from build123d import *

# Parameters (mm, degrees)
AUFSATZ_LINEAR_AUSTRAGEN1_DEPTH = 20
AUFSATZ_LINEAR_AUSTRAGEN2_DEPTH = 10
SKIZZE3_R                       = 25
SCHNITT_LINEAR_AUSTRAGEN1_DEPTH = 15


with BuildPart() as part:
    # Skizze1 → Aufsatz-Linear austragen1 (new body)
    with BuildSketch(Plane.XY):
        with BuildLine():
            Line((-0.330334949, 95.09360025), (369.669665051, 95.09360025))
            ThreePointArc((369.669665051, 95.09360025), (405.02500411, 80.448939309), (419.669665051, 45.09360025))
            Line((419.669665051, 45.09360025), (419.669665051, -224.90639975))
            ThreePointArc((419.669665051, -224.90639975), (405.02500411, -260.26173881), (369.669665051, -274.90639975))
            Line((369.669665051, -274.90639975), (-0.330334949, -274.90639975))
            ThreePointArc((-0.330334949, -274.90639975), (-35.685674008, -260.26173881), (-50.330334949, -224.90639975))
            Line((-50.330334949, -224.90639975), (-50.330334949, 45.09360025))
            ThreePointArc((-50.330334949, 45.09360025), (-35.685674008, 80.448939309), (-0.330334949, 95.09360025))
        make_face()
        with BuildLine():
            Line((-0.330334949, 85.09360025), (369.669665051, 85.09360025))
            ThreePointArc((369.669665051, 85.09360025), (397.953936298, 73.377871497), (409.669665051, 45.09360025))
            Line((409.669665051, 45.09360025), (409.669665051, -224.90639975))
            ThreePointArc((409.669665051, -224.90639975), (397.953936298, -253.190670998), (369.669665051, -264.90639975))
            Line((369.669665051, -264.90639975), (-0.330334949, -264.90639975))
            ThreePointArc((-0.330334949, -264.90639975), (-28.614606196, -253.190670998), (-40.330334949, -224.90639975))
            Line((-40.330334949, -224.90639975), (-40.330334949, 45.09360025))
            ThreePointArc((-40.330334949, 45.09360025), (-28.614606196, 73.377871497), (-0.330334949, 85.09360025))
        make_face(mode=Mode.SUBTRACT)
    extrude(amount=AUFSATZ_LINEAR_AUSTRAGEN1_DEPTH)

    # Skizze2 → Aufsatz-Linear austragen2 (add)
    with BuildSketch(Plane.XY):
        with BuildLine():
            Line((-0.330334949, -264.90639975), (369.669665051, -264.90639975))
            ThreePointArc((369.669665051, -264.90639975), (397.953936298, -253.190670998), (409.669665051, -224.90639975))
            Line((409.669665051, -224.90639975), (409.669665051, 45.09360025))
            ThreePointArc((409.669665051, 45.09360025), (397.953936298, 73.377871497), (369.669665051, 85.09360025))
            Line((369.669665051, 85.09360025), (-0.330334949, 85.09360025))
            ThreePointArc((-0.330334949, 85.09360025), (-28.614606196, 73.377871497), (-40.330334949, 45.09360025))
            Line((-40.330334949, 45.09360025), (-40.330334949, -224.90639975))
            ThreePointArc((-40.330334949, -224.90639975), (-28.614606196, -253.190670998), (-0.330334949, -264.90639975))
        make_face()
    extrude(amount=AUFSATZ_LINEAR_AUSTRAGEN2_DEPTH)

    # Skizze3 → Schnitt-Linear austragen1 (cut)
    with BuildSketch(Plane.XY):
        with Locations((184.669665051, -34.90639975)):
            Circle(SKIZZE3_R)
    extrude(amount=SCHNITT_LINEAR_AUSTRAGEN1_DEPTH, mode=Mode.SUBTRACT)


solid = part.part
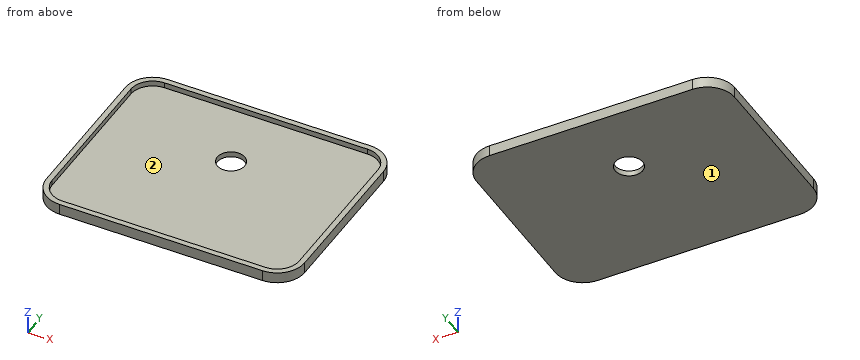
Input: part model. Units: mm. Frame: model coordinates. Face numbers are marked on the shaded views. Round coordinates to 2 decimals unless told otherwise and drop trailing zeros. Order: outer loops, then holes, each group sorted by start corner. A loop starts at its lowest first (then second) coordinate and runs counter-clockwise, first axis right, second up.
1. Cut plane B-B, the plane x = 85. Output: boundary loops of the cut face in (y, z), then the cut area to 3 significant figures.
The answers:
outline: (-274.91, 0) - (95.09, 0) - (95.09, 20) - (85.09, 20) - (85.09, 10) - (-264.91, 10) - (-264.91, 20) - (-274.91, 20) - close
area: 3,900 mm2
2. Mould query, pull axis Y, two halves, no side actions, for the marked faces 1 and 2. Classes: released by +Y, released by -Y, zero draft, split by the parting line, or undercut.
The answers:
face 1: zero draft
face 2: undercut
3. Material intervals for line 1 (X direction, y = -224, z = 14); line 2 (Y direction, x = 276, z = 12.25); line 3 (X direction, y = 46, z = 5.75), sorted ascending.
The answers:
line 1: x = -50.33 to -40.33, 409.67 to 419.67
line 2: y = -274.91 to -264.91, 85.09 to 95.09
line 3: x = -50.32 to 419.66
4. Pin query (flat end, axial travel): P1, Ø4, axis at x = 209.5, y = -203, coming from the +Z side. Return the tip coordinate at first contact, or that it passes through.
The answers:
P1: stops at z = 10
5. Cut plane A-A, the plane z = 16.75. Output: boundary loops of the cut face in (x, y), then the cut area to 3 significant figures.
The answers:
outline: (-50.33, -224.91) arc R50 ccw to (-0.33, -274.91) - (369.67, -274.91) arc R50 ccw to (419.67, -224.91) - (419.67, 45.09) arc R50 ccw to (369.67, 95.09) - (-0.33, 95.09) arc R50 ccw to (-50.33, 45.09) - close; hole (-40.33, -224.91) arc R40 ccw to (-0.33, -264.91) - (369.67, -264.91) arc R40 ccw to (409.67, -224.91) - (409.67, 45.09) arc R40 ccw to (369.67, 85.09) - (-0.33, 85.09) arc R40 ccw to (-40.33, 45.09) - close
area: 15,600 mm2
6. Cut plane C-C, the plane y = -80.5. Output: boundary loops of the cut face in (x, z), then the cut area to 3 significant figures.
The answers:
outline: (-50.33, 0) - (419.67, 0) - (419.67, 20) - (409.67, 20) - (409.67, 10) - (-40.33, 10) - (-40.33, 20) - (-50.33, 20) - close
area: 4,900 mm2
